Model file for the job. Use its own axes, mm. A direction names the side the tool comes from. Give positions to 0.01 mm unless a question says otherwise; leave off trailing zeros. Loops run counter-clockwise (first coordinate to the right, second up) from the corner with the lowest first, then second, coordinate; pieces in that order, holes last. Notation, with made-up numbers: (16.5, 67.25) - (51.5, 67.25) arc R25 cw to (51.5, 97.25) - close; hole circle Ø2 at (71, -14.5). An arc over 180 degrees is marked (long way). Use a Markdown table: item, result.
from build123d import *

# Parameters (mm, degrees)
SALIENTE_EXTRUIR1_DEPTH = 8.5
CROQUIS2_R              = 12
SALIENTE_EXTRUIR2_DEPTH = 27.4
CROQUIS3_R              = 5
CORTAR_EXTRUIR1_DEPTH   = 35.9
CROQUIS4_R              = 8.5
CORTAR_EXTRUIR2_DEPTH   = 1
CROQUIS5_R              = 8.5
CORTAR_EXTRUIR3_DEPTH   = 1
CROQUIS6_R              = 2.25
CORTAR_EXTRUIR4_DEPTH   = 8.5


with BuildPart() as part:
    # Croquis1 → Saliente-Extruir1 (new body)
    with BuildSketch(Plane.XY):
        with BuildLine():
            Line((-13.228756555, 15), (13.228756555, 15))
            ThreePointArc((13.228756555, 15), (20, 0), (13.228756555, -15))
            Line((13.228756555, -15), (-13.228756555, -15))
            ThreePointArc((-13.228756555, -15), (-20, 0), (-13.228756555, 15))
        make_face()
    extrude(amount=SALIENTE_EXTRUIR1_DEPTH)

    # Croquis2 → Saliente-Extruir2 (add)
    with BuildSketch(Plane.XY.offset(8.5)):
        Circle(CROQUIS2_R)
    extrude(amount=SALIENTE_EXTRUIR2_DEPTH)

    # Croquis3 → Cortar-Extruir1 (cut)
    with BuildSketch(Plane.XY.offset(35.9)):
        Circle(CROQUIS3_R)
    extrude(amount=-CORTAR_EXTRUIR1_DEPTH, mode=Mode.SUBTRACT)

    # Croquis4 → Cortar-Extruir2 (cut)
    with BuildSketch(Plane.XY.offset(35.9)):
        Circle(CROQUIS4_R)
    extrude(amount=-CORTAR_EXTRUIR2_DEPTH, mode=Mode.SUBTRACT)

    # Croquis5 → Cortar-Extruir3 (cut)
    with BuildSketch(Plane(origin=(0, 0, 0), x_dir=(-1, 0, 0), z_dir=(0, 0, -1))):
        Circle(CROQUIS5_R)
    extrude(amount=-CORTAR_EXTRUIR3_DEPTH, mode=Mode.SUBTRACT)

    # Croquis6 → Cortar-Extruir4 (cut)
    with BuildSketch(Plane(origin=(0, 0, 0), x_dir=(-1, 0, 0), z_dir=(0, 0, -1))):
        with Locations((11.37991652, -11.6)):
            Circle(CROQUIS6_R)
        with Locations((16.25, 0)):
            Circle(CROQUIS6_R)
        with Locations((11.37991652, 11.6)):
            Circle(CROQUIS6_R)
        with Locations((-11.37991652, -11.6)):
            Circle(CROQUIS6_R)
        with Locations((-16.25, 0)):
            Circle(CROQUIS6_R)
        with Locations((-11.37991652, 11.6)):
            Circle(CROQUIS6_R)
    extrude(amount=-CORTAR_EXTRUIR4_DEPTH, mode=Mode.SUBTRACT)


solid = part.part
(1) Slice it at D-D, the plane y = -10. Write the cut outline in (x, z).
Computed:
| item | result |
|---|---|
| outline | (-17.32, 0) - (-12.96, 0) - (-12.96, 8.5) - (-17.32, 8.5) - close; (-9.8, 0) - (9.8, 0) - (9.8, 8.5) - (6.63, 8.5) - (6.63, 35.9) - (-6.63, 35.9) - (-6.63, 8.5) - (-9.8, 8.5) - close; (12.96, 0) - (17.32, 0) - (17.32, 8.5) - (12.96, 8.5) - close |
(2) Slice it at C-C, the plane x = 3.5. Write the cut outline in (y, z).
Computed:
| item | result |
|---|---|
| outline | (-15, 0) - (-7.75, 0) - (-7.75, 1) - (-3.57, 1) - (-3.57, 34.9) - (-7.75, 34.9) - (-7.75, 35.9) - (-11.48, 35.9) - (-11.48, 8.5) - (-15, 8.5) - close; (3.57, 1) - (7.75, 1) - (7.75, 0) - (15, 0) - (15, 8.5) - (11.48, 8.5) - (11.48, 35.9) - (7.75, 35.9) - (7.75, 34.9) - (3.57, 34.9) - close |
(3) Slice it at B-B, the plane z = 8. Write the cut outline in (x, y), plus the area to 3 significant figures.
Computed:
| item | result |
|---|---|
| outline | (-13.23, -15) - (13.23, -15) arc R20 ccw to (13.23, 15) - (-13.23, 15) arc R20 ccw to start; hole circle Ø4.5 at (-16.25, 0); hole circle Ø4.5 at (-11.38, -11.6); hole circle Ø4.5 at (-11.38, 11.6); hole circle Ø10 at (0, 0); hole circle Ø4.5 at (11.38, -11.6); hole circle Ø4.5 at (11.38, 11.6); hole circle Ø4.5 at (16.25, 0) |
| area | 901 mm² |
(4) Drill centre lines: probe 1 along Z at (x, y) = (13, 6); probe 2 along Z at (x, y) = (0, 6.75); probe 3 along Y at (x, z) = (0, 23.5). Where is each one in solid material? Low to high. Write a range as [from, to].
Computed:
| item | result |
|---|---|
| probe 1 | [0, 8.5] |
| probe 2 | [1, 34.9] |
| probe 3 | [-12, -5], [5, 12] |
(5) Slice it at A-A, the plane y = 0. Write the cut outline in (x, z), plus the area to 3 significant figures.
Computed:
| item | result |
|---|---|
| outline | (-20, 0) - (-18.5, 0) - (-18.5, 8.5) - (-20, 8.5) - close; (-14, 0) - (-8.5, 0) - (-8.5, 1) - (-5, 1) - (-5, 34.9) - (-8.5, 34.9) - (-8.5, 35.9) - (-12, 35.9) - (-12, 8.5) - (-14, 8.5) - close; (5, 1) - (8.5, 1) - (8.5, 0) - (14, 0) - (14, 8.5) - (12, 8.5) - (12, 35.9) - (8.5, 35.9) - (8.5, 34.9) - (5, 34.9) - close; (18.5, 0) - (20, 0) - (20, 8.5) - (18.5, 8.5) - close |
| area | 548 mm² |
(6) Mould opens along Y. For faces 4 (the cylindrical face through (-20, 0, 4)), 5 (the flat face through (-8.2, 2.8, 35.9)), 6 (the cylindrical face through (-12.418, 9.604, 4.19)), 7 (the cylindrical face through (4.57, 7.167, 35.407)) say: pulls with the +Y half, pulls with the -Y half, needs draft (parallel to the pull), parting line crosses it, or undercut.
Computed:
| item | result |
|---|---|
| face 4 | parting line crosses it |
| face 5 | needs draft |
| face 6 | undercut |
| face 7 | undercut |
(7) 3-axis set-ups, long thin cutter, end or side, ignore diameter. For faces 1 (the cylindrical face through (-18.396, 0.676, 4.19)), 2 (the flat face through (-4, -4, 1)), 3 (the flat face through (9, -10, 8.5)): which of +Z, -Z, +X, -X, +Y, -Y reach the whole face in a straight line?
Computed:
| item | result |
|---|---|
| face 1 | +Z, -Z |
| face 2 | -Z |
| face 3 | +Z |
(8) Pin check, flat tips, straight feed: P1, Ø3, axis at y = 8, z = 7, coming from the +X side; P2, Ø12, axis at y = 1.5, z = 11.5, coming from the -X side; P3, Ø4, axis at y = -5.5, z = 32, coming from the -X side. Stop position of each tip, or through.
Computed:
| item | result |
|---|---|
| P1 | x = 18.91 |
| P2 | x = -20 |
| P3 | x = -11.48 |
